Design review of the part built by this model. Coordinates are the model's own, in mm. Face numbers are marked on the shaded views. Round coordinates to 2 decimals unless told otherwise and drop trailing zeros. Loops run counter-clockwise (first coordinate to the right, second up) from the corner with the lowest first, then second, coordinate; pieces in that order, holes last. Notation, with made-up numbers: (72, 68.25) -> (82, 68.25) arc R27 cw to (82, 88.25) -> close; hole circle Ø10 at (-5.5, 2.25). An arc over 180 degrees is marked (long way). Use a Markdown table: item, result. Add a question column.
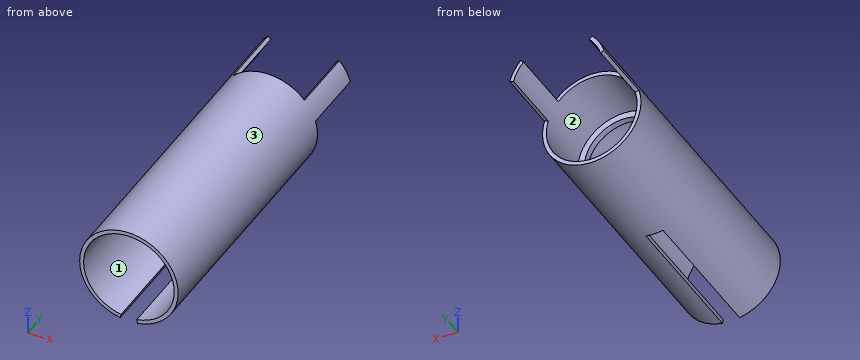
Autodesk Inventor part; units mm, degrees
ref_plane "YZ Plane" through (0, 0, 0) normal (1, 0, 0) x (0, 1, 0)
ref_plane "XZ Plane" through (0, 0, 0) normal (0, 1, 0) x (-1, 0, 0)
ref_plane "XY Plane" through (0, 0, 0) normal (0, 0, 1) x (1, 0, 0)
sketch "スケッチ1" plane through (0, 0, 0) normal (0, 1, 0) x (-1, 0, 0)
  circle A0 centre (0, 0) radius 35
  circle A1 centre (0, 0) radius 38
  dimension "d0" = 70
  dimension "d1" = 76
extrude "押し出し1" add sketch "スケッチ1" along normal blind 250
sketch "スケッチ2" plane through (0, 250, 0) normal (0, 1, 0) x (1, 0, 0)
  circle A0 centre (0, 0) radius 38
  line L0 (0, 0) -> (-27.1351, -26.6024)
  line L1 (0, 0) -> (27.9749, -25.7178)
  line L2 (0, 0) -> (-27.1351, -26.6024)
  circle A1 centre (0, 0) radius 35
  line L3 (0, 0) -> (-36.4384, -10.7818)
  line L4 (0, 0) -> (36.4384, -10.7818)
  point P0 (-32.2602, -20.0818)
  point P1 (33.0208, -18.805)
extrude "押し出し3" cut sketch "スケッチ2" against normal blind 50 contours A0 L4 A1 L3 | L0 A1 L1 A0 | A1 L4 L3 | L0 L1 A1
ref_plane "作業平面2" through (0, 150, 0) normal (0, -1, 0) x (1, 0, 0)
sketch "スケッチ3" plane through (0, 150, 0) normal (0, -1, 0) x (1, 0, 0)
  circle A0 centre (0, 0) radius 35
  circle A1 centre (0, 0) radius 30
  dimension "d10" = 70
  dimension "d11" = 60
extrude "押し出し4" add sketch "スケッチ3" against normal blind 5
sketch "スケッチ4" plane through (0, 0, 0) normal (0, -1, 0) x (1, 0, 0)
  circle A0 centre (0, 0) radius 38
  line L0 (0, 0) -> (6.5986, -37.4227)
  line L1 (0, 0) -> (38, 0) construction
  line L2 (0, 0) -> (-6.5986, -37.4227)
  line L3 (0, 0) -> (38, 0) construction
  dimension "d14" = 80
  dimension "d15" = 100
extrude "押し出し5" cut sketch "スケッチ4" against normal blind 110 contours L2 L0 A0 picked at (0, -25.2905)
properties part number "知能ロボコン大砲１"
1. To check wall thickness, follow probe 1 along X at (y, z) = (96.5, 0); probe 2 along Z at (x, y) = (0, 151). State the ranges of each line that lie inside material, in increasing order. Write a range as from..to.
2. Consider section D-D on y = 89.5. State the section outline as (x, z) points.
3. Mouldability with a two-part tool opening along Z and no side actions: class the marked faces 1, 2 and 3 as +Z half, -Z half, draft (parallel to the pull), parting line (faces both ways), or undercut.
4. Consider section C-C on y = 163. State the section outline as (x, z) points, plus the area to 3 significant figures.
5. Consider section A-A on x = 0. State the section outline as (y, z) points.
6. Consider section B-B on z = 0. State the section outline as (x, y) points, plus the area to 3 significant figures.
7. Insertion check: P1, Ø15.5, axis at x = -12, z = 32, coming from the +Y side; P2, Ø6, axis at x = -24.5, y = 194.5, coming from the -Z side; P3, Ø8, axis at x = -23.5, y = 217.5, coming from the +Z side; P4, Ø24.5, axis at x = 14, z = -3.5, coming from the +Y side. Each pin has a flat end and moves straight along its axis. Give the tip position at first contact, or say it passes through.
Verdict:
| question | item | result |
|---|---|---|
| 1 | probe 1 | x = -38..-35, 35..38 |
| 1 | probe 2 | z = -38..-30, 30..38 |
| 2 | outline | (-6.6, -37.42) -> (-6.08, -34.47) arc R35 cw (long way) to (6.08, -34.47) -> (6.6, -37.42) arc R38 ccw (long way) to start |
| 3 | face 1 | undercut |
| 3 | face 2 | undercut |
| 3 | face 3 | parting line |
| 4 | outline | circle Ø76 at (0, 0); hole circle Ø70 at (0, 0) |
| 4 | area | 688 mm² |
| 5 | outline | (0, 35) -> (150, 35) -> (150, 30) -> (155, 30) -> (155, 35) -> (200, 35) -> (200, 38) -> (0, 38) -> close; (110, -38) -> (200, -38) -> (200, -35) -> (155, -35) -> (155, -30) -> (150, -30) -> (150, -35) -> (110, -35) -> close |
| 6 | outline | (-38, 0) -> (-35, 0) -> (-35, 150) -> (-30, 150) -> (-30, 155) -> (-35, 155) -> (-35, 200) -> (-38, 200) -> close; (30, 150) -> (35, 150) -> (35, 0) -> (38, 0) -> (38, 200) -> (35, 200) -> (35, 155) -> (30, 155) -> close |
| 6 | area | 1,250 mm² |
| 7 | P1 | stops at y = 200 |
| 7 | P2 | stops at z = -31.33 |
| 7 | P3 | stops at z = 26.6 |
| 7 | P4 | passes through |
